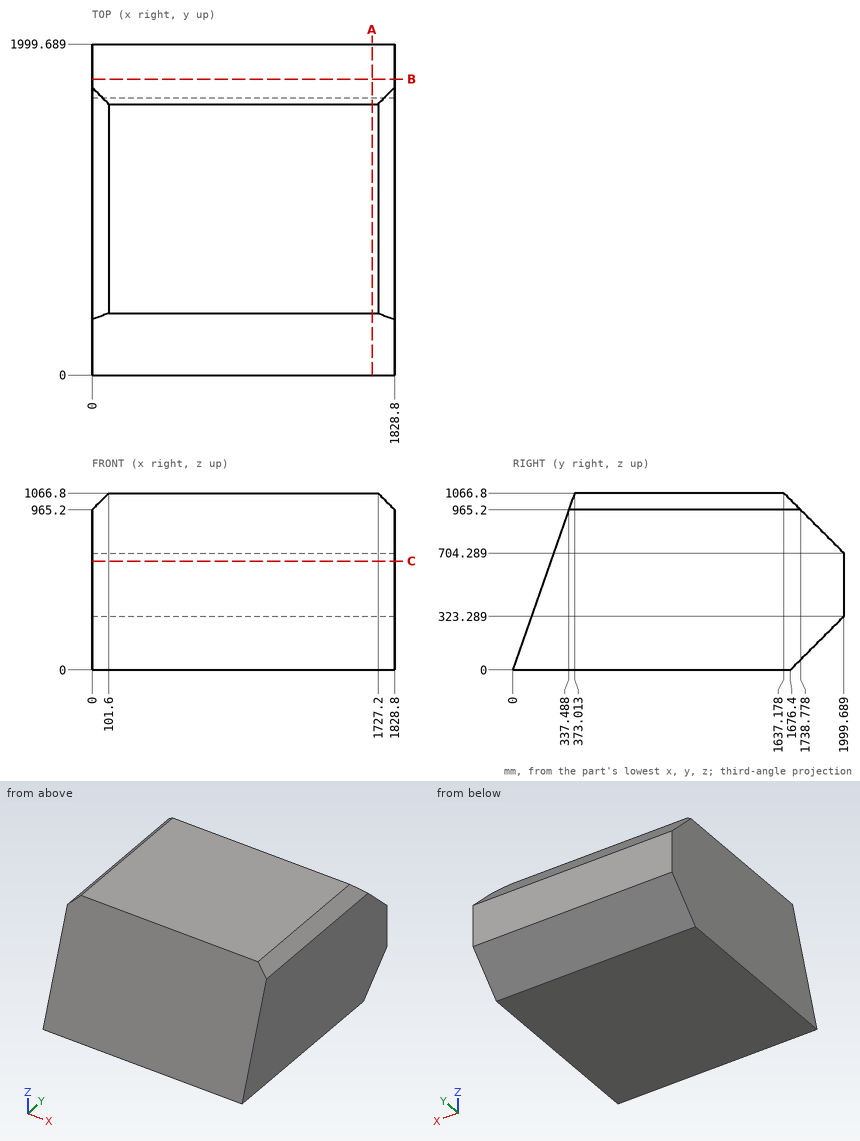
Drawing for the job (mm, zero at the part's lowest x, y, z). Coordinates: 2 decimals unless noted, no trailing zeros. Write each loop counter-clockwise with the first axis right and the second up, starting at its lowest first coordinate (ties: lowest second). Pieces come first, ordered by that corner, then holes. Notation, with made-up numbers: (6.25, -30.75) -> (59.25, -30.75) arc R30 ccw to (59.25, -3.75) -> close; hole circle Ø6 at (18, 77). An arc over 180 degrees is marked (long way). One line per item, written item: value. Start each with the question number.
1) Flat gauge pins, fed straight in: pin 1 Ø5 at (x, z) = (437, 896) entering from +Y; pin 2 Ø1.5 at (x, y) = (681.5, 1760.5) entering from -Z. Where does each tip first touch, or does it go through?
2) Slice it at B-B on y = 1787.5. Write the cut outline in (x, z), then the cut area to 3 significant figures.
3) Slice it at C-C on z = 656. Write the cut outline in (x, y), then the cut area to 3 significant figures.
4) Probe probe 1 along Y at (x, z) = (1010, 590); probe 2 along Z at (x, y) = (1742.5, 667.5); probe 3 along Y at (x, z) = (413, 599) (1 decimal). List the from-to ranges inside material, lowest first.
5) Slice it at A-A on x = 1692. Write the cut outline in (y, z), then the cut area to 3 significant figures.
Answers follow:
1. pin 1: y = 1810.48
1. pin 2: z = 83.35
2. outline: (0, 111.1) -> (1828.8, 111.1) -> (1828.8, 916.48) -> (0, 916.48) -> close
2. area: 1,470,000 mm2
3. outline: (0, 229.37) -> (1828.8, 229.37) -> (1828.8, 1999.69) -> (0, 1999.69) -> close
3. area: 3,240,000 mm2
4. probe 1: 206.3 to 1999.69
4. probe 2: 0 to 1051.5
4. probe 3: 209.4 to 1999.7
5. outline: (0, 0) -> (1676.4, 0) -> (1999.69, 323.29) -> (1999.69, 704.29) -> (1637.18, 1066.8) -> (373.01, 1066.8) -> close
5. area: 1,820,000 mm2
